Source: CAD feature listing. Evaluate the final solid. Frame: model axes, mm. Round coordinates to 2 decimals unless told otherwise and drop trailing zeros. Write each loop counter-clockwise with the first axis right and the second up, starting at its lowest first coordinate (ties: lowest second). Pieces come first, ordered by that corner, then holes.
from build123d import *

# Parameters (mm, degrees)
SKETCH_1_R               = 5
SKETCH_1_R_2             = 4
EXTRUDE_1_DEPTH          = 124.5
SKETCH_2_R               = 2
CUT_EXTRUDE_1_DEPTH      = 6
CUT_EXTRUDE_1_DEPTH_BACK = 6


with BuildPart() as part:
    # 草图1 → 拉伸-薄壁1 (new body, symmetric)
    with BuildSketch(Plane(origin=(0, 0, 0), x_dir=(1, 0, 0), z_dir=(0, 1, 0))):
        Circle(SKETCH_1_R)
        Circle(SKETCH_1_R_2, mode=Mode.SUBTRACT)
    extrude(amount=EXTRUDE_1_DEPTH, both=True)

    # 草图2 → 切除-拉伸1 (cut, two sides)
    with BuildSketch(Plane.XY) as cut_extrude_1_sk:
        with Locations((0, -107.5)):
            Circle(SKETCH_2_R)
        with Locations((0, 107.5)):
            Circle(SKETCH_2_R)
    extrude(amount=CUT_EXTRUDE_1_DEPTH, mode=Mode.SUBTRACT)
    extrude(cut_extrude_1_sk.sketch, amount=-CUT_EXTRUDE_1_DEPTH_BACK, mode=Mode.SUBTRACT)


solid = part.part
1) Section query C-C on y = 100. Return the cut outline in (x, z).
Taken from the geometry:
outline: circle Ø10 at (0, 0); hole circle Ø8 at (0, 0)
2) Section query A-A on z = 0. Return the cut outline in (x, y).
Taken from the geometry:
outline: (-5, -124.5) - (-4, -124.5) - (-4, 124.5) - (-5, 124.5) - close; (4, -124.5) - (5, -124.5) - (5, 124.5) - (4, 124.5) - close
3) Pull-direction query (X, two-part tool) for faces 1 (the face through (-1.998, -107.412, 4.223)), 2 (the face through (3.695, -1.743, 1.532)), 3 (the face through (4.619, 1.743, 1.915)); classes: released by +X, released by -X, zero draft, split by the parting line, or undercut.
Taken from the geometry:
face 1: undercut
face 2: undercut
face 3: split by the parting line
4) Section query D-D on y = -107.5. Return the cut outline in (x, z).
Taken from the geometry:
outline: (-2, -4.58) - (-2, -3.46) arc R4 cw to (-2, 3.46) - (-2, 4.58) arc R5 ccw to start; (2, -4.58) arc R5 ccw to (2, 4.58) - (2, 3.46) arc R4 cw to (2, -3.46) - close
5) Contact query for flat-ended pins moving along their axis: P1, Ø1.5, axis at x = 3, y = 37.5, coming from the +Z side; P2, Ø5, axis at x = 3, y = 48, coming from the -Z side. Output: stop coordinate, or through.
Taken from the geometry:
P1: stops at z = 4.47
P2: stops at z = -4.97
6) Section query B-B on x = 0. Return the cut outline in (y, z).
Taken from the geometry:
outline: (-124.5, -5) - (-109.5, -5) - (-109.5, -4) - (-124.5, -4) - close; (-124.5, 4) - (-109.5, 4) - (-109.5, 5) - (-124.5, 5) - close; (-105.5, -5) - (105.5, -5) - (105.5, -4) - (-105.5, -4) - close; (-105.5, 4) - (105.5, 4) - (105.5, 5) - (-105.5, 5) - close; (109.5, -5) - (124.5, -5) - (124.5, -4) - (109.5, -4) - close; (109.5, 4) - (124.5, 4) - (124.5, 5) - (109.5, 5) - close
7) Material intervals for line 1 (Y direction, x = 0, z = -4.5); line 2 (Z direction, x = -0.25, y = 97); line 3 (X direction, y = 36.5, z = 0.75), sorted ascending.
Taken from the geometry:
line 1: y = -124.5 to -109.5, -105.5 to 105.5, 109.5 to 124.5
line 2: z = -4.99 to -3.99, 3.99 to 4.99
line 3: x = -4.94 to -3.93, 3.93 to 4.94
